Source: CAD feature listing. Evaluate the final solid. Frame: model axes, mm. Face numbers are marked on the shaded views. Give positions to 0.01 mm unless a question says otherwise; leave off trailing zeros. Order: outer loops, then holes, each group sorted by start corner. A loop starts at its lowest first (then second) coordinate and runs counter-clockwise, first axis right, second up.
1) Section C-C, the plane z = 29. Return loops of the section in (x, y), plus the area to 3 significant figures.
2) Draft query along Y for the marked faces 1, 2, 3 and 4. Return one class per face: released by +Y, released by -Y, zero draft, split by the parting line, or undercut.
3) Section B-B, the plane y = -30.5. Return loops of the section in (x, z), plus the area to 3 significant figures.
4) Material intervals for line 1 (Y direction, x = -46.3, z = 48.1); line 2 (Y direction, x = 80, z = 47.45); line 3 (Y direction, x = -46, z = 47), sorted ascending.
5) Section A-A, the plane x = 87. Return loops of the section in (y, z).
6) Section D-D, the plane y = 29. Return loops of the section in (x, z), plus the area to 3 significant figures.
7) First-contact query: P1, Ø2.5, axis at x = -78, z = 47, coming from the -Y side (3 decimals); P2, Ø3, axis at x = -80.5, z = 33, coming from the +Y side; P3, Ø12, axis at y = 16, z = 5, coming from the +X side; P4, Ø2.5, axis at x = -31.7, y = -51.56, coming from the -Z side. Flat tips, straight axial feed; report the tip coordinate or a pass-through.
```python
from build123d import *

# Parameters (mm, degrees)
ESQUISSE1_R             = 105
BOSS_EXTRU_1_DEPTH      = 50
COQUE1_T                = -5
ESQUISSE3_R             = 25
ESQUISSE3_R_2           = 1.5
ENL_V_MAT_EXTRU_1_DEPTH = 10
ENL_V_MAT_EXTRU_2_DEPTH = 156.161206492
ENL_V_MAT_EXTRU_3_DEPTH = 45
ESQUISSE7_R             = 1.5
ENL_V_MAT_EXTRU_4_DEPTH = 156.161206492
ESQUISSE8_W             = 11
ESQUISSE8_H             = 31.895350387
ENL_V_MAT_EXTRU_5_DEPTH = 5
ESQUISSE9_R             = 15.5
ENL_V_MAT_EXTRU_7_DEPTH = 156.161206492
BALAYAGE1_PROFILE_R     = 1.5
BOSS_EXTRU_2_START      = 1
BOSS_EXTRU_2_DEPTH      = 1
BALAYAGE2_PROFILE_R     = 1.5
BOSS_EXTRU_3_START      = 2
BOSS_EXTRU_3_DEPTH      = 2
ESQUISSE30_R            = 1.5
BOSS_EXTRU_4_DEPTH      = 5
ESQUISSE31_R            = 12
ENL_V_MAT_EXTRU_8_DEPTH = 5


with BuildPart() as part:
    # Esquisse1 → Boss.-Extru.1 (new body)
    with BuildSketch(Plane.XY):
        Circle(ESQUISSE1_R)
    extrude(amount=BOSS_EXTRU_1_DEPTH)

    # Coque1
    coque1_openings = [part.faces().sort_by_distance(p)[0] for p in [
        (0, 0, 0),
    ]]
    offset(amount=COQUE1_T, openings=coque1_openings, kind=Kind.INTERSECTION)

    # Esquisse3 → Enlèv. mat.-Extru.1 (cut)
    with BuildSketch(Plane(origin=(0, 0, 45), x_dir=(-1, 0, 0), z_dir=(0, 0, -1))):
        with Locations((-3.8, -24.557615642)):
            Circle(ESQUISSE3_R)
        with Locations((-23.669465397, 4.134521322)):
            Circle(ESQUISSE3_R_2)
        with Locations((16.069465397, 4.134521322)):
            Circle(ESQUISSE3_R_2)
        with Locations((31.7, -51.557615642)):
            Circle(ESQUISSE3_R_2)
    extrude(amount=-ENL_V_MAT_EXTRU_1_DEPTH, mode=Mode.SUBTRACT)

    # Esquisse5 → Enlèv. mat.-Extru.2 (cut, through all)
    with BuildSketch(Plane(origin=(0, 0, 45), x_dir=(-1, 0, 0), z_dir=(0, 0, -1))):
        with BuildLine():
            Line((-42.388918531, 10.472597699), (35.07440103, 10.472597699))
            ThreePointArc((35.07440103, 10.472597699), (37.195721374, 11.351277356), (38.07440103, 13.472597699))
            Line((38.07440103, 13.472597699), (38.07440103, 45.806945365))
            ThreePointArc((38.07440103, 45.806945365), (37.195721374, 47.928265708), (35.07440103, 48.806945365))
            Line((35.07440103, 48.806945365), (-42.388918531, 48.806945365))
            ThreePointArc((-42.388918531, 48.806945365), (-44.510238875, 47.928265708), (-45.388918531, 45.806945365))
            Line((-45.388918531, 45.806945365), (-45.388918531, 13.472597699))
            ThreePointArc((-45.388918531, 13.472597699), (-44.510238875, 11.351277356), (-42.388918531, 10.472597699))
        make_face()
    extrude(amount=-ENL_V_MAT_EXTRU_2_DEPTH, mode=Mode.SUBTRACT)

    # Esquisse6 → Enlèv. mat.-Extru.3 (cut)
    with BuildSketch(Plane(origin=(0, 0, 0), x_dir=(-1, 0, 0), z_dir=(0, 0, -1))):
        with BuildLine():
            Line((-78.81072608, -69.38205427), (78.81072608, -69.38205427))
            ThreePointArc((78.81072608, -69.38205427), (0, -105), (-78.81072608, -69.38205427))
        make_face()
    extrude(amount=-ENL_V_MAT_EXTRU_3_DEPTH, mode=Mode.SUBTRACT)

    # Esquisse7 → Enlèv. mat.-Extru.4 (cut, through all)
    with BuildSketch(Plane(origin=(0, 0, 45), x_dir=(-1, 0, 0), z_dir=(0, 0, -1))):
        with Locations((52.614229855, 48.990085475)):
            Circle(ESQUISSE7_R)
        with Locations((52.614229855, 11.990085475)):
            Circle(ESQUISSE7_R)
        with Locations((46.3, -26.057615642)):
            Circle(ESQUISSE7_R)
        with Locations((46.3, -53.057615642)):
            Circle(ESQUISSE7_R)
        with Locations((-46.3, -26.062213408)):
            Circle(ESQUISSE7_R)
        with Locations((-46.3, -53.062213408)):
            Circle(ESQUISSE7_R)
    extrude(amount=-ENL_V_MAT_EXTRU_4_DEPTH, mode=Mode.SUBTRACT)

    # Esquisse8 → Enlèv. mat.-Extru.5 (cut)
    with BuildSketch(Plane(origin=(0, 0, 45), x_dir=(-1, 0, 0), z_dir=(0, 0, -1))):
        with Locations((-75.3, -39.589403314)):
            Rectangle(ESQUISSE8_W, ESQUISSE8_H)
        with Locations((75.3, -39.589403314)):
            Rectangle(ESQUISSE8_W, ESQUISSE8_H)
    extrude(amount=-ENL_V_MAT_EXTRU_5_DEPTH, mode=Mode.SUBTRACT)

    # Esquisse9 → Enlèv. mat.-Extru.7 (cut, through all)
    with BuildSketch(Plane(origin=(0, 0, 45), x_dir=(-1, 0, 0), z_dir=(0, 0, -1))):
        with Locations((34.681880454, 70.440085475)):
            Circle(ESQUISSE9_R)
        with Locations((-34.681880454, 70.440085475)):
            Circle(ESQUISSE9_R)
    extrude(amount=-ENL_V_MAT_EXTRU_7_DEPTH, mode=Mode.SUBTRACT)

    # Balayage1: sweep along a path in Esquisse10
    with BuildLine(Plane(origin=(-9.681880454, 0.440085475, 22), x_dir=(-1, 0, 0), z_dir=(0, 0, -1))) as balayage1_path:
        Line((-43.221417057, 88.965628134), (-42.925873334, 93.872357698))
    # Balayage1 profile (on start of the path) → Balayage1 (sweep)
    with BuildSketch(Plane(origin=(33.539536603, 89.405713609, 22), x_dir=(0.9981909544337458, 0.060123360573471965, 0), z_dir=(-0.060123360573471965, 0.9981909544337458, 0))):
        Circle(BALAYAGE1_PROFILE_R)
    balayage1 = sweep(path=balayage1_path.line)

    # Esquisse19 → Boss.-Extru.2 (add)
    with BuildSketch(Plane(origin=(-5.53995205, 91.976396052, 0), x_dir=(0.998190954433746, 0.06012336057346903, 0), z_dir=(-0.06012336057346903, 0.998190954433746, 0)).offset(BOSS_EXTRU_2_START)):
        with BuildLine():
            Line((38.85423401, -23.5), (38.85423401, -20.5))
            ThreePointArc((38.85423401, -20.5), (37.35423401, -22), (38.85423401, -23.5))
        make_face()
    boss_extru_2 = extrude(amount=-BOSS_EXTRU_2_DEPTH)

    # Balayage2: sweep along a path in Esquisse20
    with BuildLine(Plane(origin=(-9.681880454, 0.440085475, 22), x_dir=(-1, 0, 0), z_dir=(0, 0, -1))) as balayage2_path:
        Line((-73.311298587, 71.743577457), (-78.469516131, 72.142702967))
    # Balayage2 profile (on start of the path) → Balayage2 (sweep)
    with BuildSketch(Plane(origin=(63.629418133, 72.183662932, 22), x_dir=(-0.07714603625431019, 0.9970198037603109, 0), z_dir=(0.9970198037603109, 0.07714603625431019, 0))):
        Circle(BALAYAGE2_PROFILE_R)
    balayage2 = sweep(path=balayage2_path.line)

    # Esquisse27 → Boss.-Extru.3 (add)
    with BuildSketch(Plane(origin=(73.961032209, 5.722855705, 0), x_dir=(0, 0, -1), z_dir=(0.9970198037603113, 0.07714603625430425, 0)).offset(BOSS_EXTRU_3_START)):
        with BuildLine():
            Line((-20.5, 67.059784053), (-23.5, 67.059784053))
            ThreePointArc((-23.5, 67.059784053), (-22, 65.559784053), (-20.5, 67.059784053))
        make_face()
    boss_extru_3 = extrude(amount=-BOSS_EXTRU_3_DEPTH)

    # Symétrie1: Balayage1, Boss.-Extru.2, Balayage2, Boss.-Extru.3 across plane
    add(balayage1.mirror(Plane(origin=(0, 0, 0), x_dir=(0, 0, 1), z_dir=(1, 0, 0))))
    add(boss_extru_2.mirror(Plane(origin=(0, 0, 0), x_dir=(0, 0, 1), z_dir=(1, 0, 0))))
    add(balayage2.mirror(Plane(origin=(0, 0, 0), x_dir=(0, 0, 1), z_dir=(1, 0, 0))))
    add(boss_extru_3.mirror(Plane(origin=(0, 0, 0), x_dir=(0, 0, 1), z_dir=(1, 0, 0))))

    # Esquisse30 → Boss.-Extru.4 (add)
    with BuildSketch(Plane(origin=(0, 0, 0), x_dir=(-1, 0, 0), z_dir=(0, 0, -1))):
        with Locations(Location((0, 102.5, 0), (0, 0, 180))):
            Circle(ESQUISSE30_R)
        with Locations(Location((-72.478445072, 72.478445072, 0), (0, 0, 180))):
            Circle(ESQUISSE30_R)
        with Locations((72.478445072, 72.478445072)):
            Circle(ESQUISSE30_R)
    extrude(amount=BOSS_EXTRU_4_DEPTH)

    # Esquisse31 → Enlèv. mat.-Extru.8 (cut)
    with BuildSketch(Plane(origin=(0, 0, 45), x_dir=(-1, 0, 0), z_dir=(0, 0, -1))):
        with Locations((-80, 25)):
            Circle(ESQUISSE31_R)
        with Locations((80, 25)):
            Circle(ESQUISSE31_R)
    extrude(amount=-ENL_V_MAT_EXTRU_8_DEPTH, mode=Mode.SUBTRACT)


solid = part.part
```
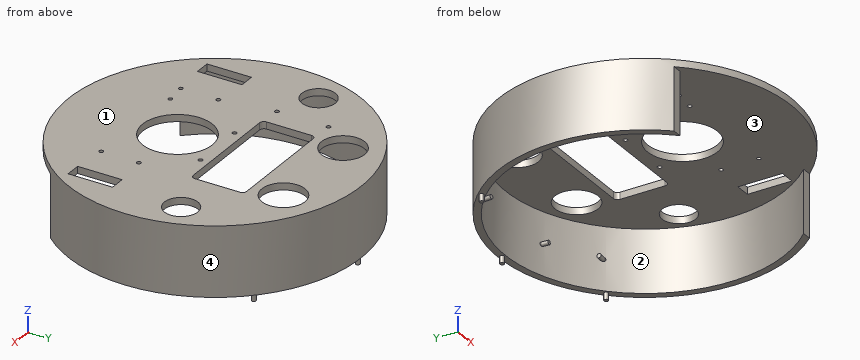
From the geometry:
1. outline: (-78.81, -69.38) - (-72.01, -69.38) arc R100 cw (long way) to (72.01, -69.38) - (78.81, -69.38) arc R105 ccw (long way) to start
1. area: 2,370 mm2
2. face 1: zero draft
2. face 2: undercut
2. face 3: undercut
2. face 4: split by the parting line
3. outline: (-100.47, 0) - (-95.24, 0) - (-95.24, 45) - (-80.8, 45) - (-80.8, 50) - (-100.47, 50) - close; (-69.8, 45) - (-20.48, 45) - (-20.48, 50) - (-69.8, 50) - close; (28.08, 45) - (69.8, 45) - (69.8, 50) - (28.08, 50) - close; (80.8, 45) - (95.24, 45) - (95.24, 0) - (100.47, 0) - (100.47, 50) - (80.8, 50) - close
3. area: 1,120 mm2
4. line 1: y = -94.24 to -54.56, -51.56 to -27.56, -24.56 to 60.18, 80.7 to 94.24
4. line 2: y = -68.01 to -55.54, -23.64 to 13, 37 to 68.01
4. line 3: y = -94.39 to -54.53, -51.59 to -27.53, -24.59 to 59.85, 81.03 to 94.39
5. outline: (-58.79, 0) - (-49.31, 0) - (-49.31, 45) - (15.25, 45) - (15.25, 50) - (-58.79, 50) - close; (34.75, 45) - (49.31, 45) - (49.31, 0) - (58.79, 0) - (58.79, 50) - (34.75, 50) - close
6. outline: (-100.92, 0) - (-95.7, 0) - (-95.7, 45) - (-91.31, 45) - (-91.31, 50) - (-100.92, 50) - close; (-68.69, 45) - (-38.07, 45) - (-38.07, 50) - (-68.69, 50) - close; (45.39, 45) - (68.69, 45) - (68.69, 50) - (45.39, 50) - close; (91.31, 45) - (95.7, 45) - (95.7, 0) - (100.92, 0) - (100.92, 50) - (91.31, 50) - close
6. area: 835 mm2
7. P1: stops at y = -71.655
7. P2: stops at y = 69.17
7. P3: stops at x = 104.52
7. P4: passes through
